Geometry check sheet. Reference: the model listing, model coordinates, mm. Face numbers are marked on the shaded views. A direction names the side the tool comes from. Round coordinates to 2 decimals unless told otherwise and drop trailing zeros. Order: outer loops, then holes, each group sorted by start corner. A loop starts at its lowest first (then second) coordinate and runs counter-clockwise, first axis right, second up. Notation, with made-up numbers: (70, 21) - (122, 21) arc R21 ccw to (122, 44) - close; hole circle Ø3 at (80, 40). An arc over 180 degrees is marked (long way). One line per question, with ' | ' between items. Start each with the question number.
Q1. Material ranges on line 1 along X through (y, z) = (-1.3, 1.25); line 2 along Z through (x, y) = (2.75, -1.25); line 3 along Z through (x, y) = (4.5, -0.45), recorded low to high.
Q2. Sectioned sample at C-C, the plane x = -0.5. Enter the section's corners in (y, z), then the cut area to 3 significant figures.
Q3. Sectioned sample at A-A, the plane y = -2. Enter the section's corners in (x, z), then the cut area to 3 significant figures.
Q4. Sectioned sample at B-B, the plane z = 2.25. Enter the section's corners in (x, y), then the cut area to 3 significant figures.
Q5. Tool access check on the marked faces 1 and 2. Record the directions out of +Z, -Z, +X, -X, +Y, -Y that give a thin tool (end or side, any length) a straight path to the whole face; none if there is none.
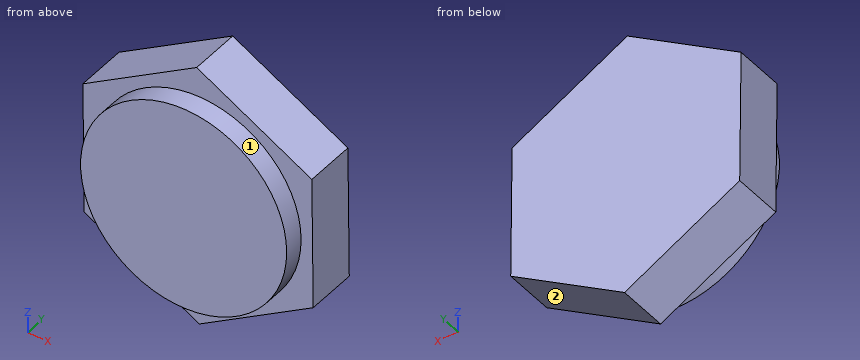
```python
from build123d import *

# Parameters (mm, degrees)
F1_DEPTH = 2.5
F2_R     = 5
F3_DEPTH = 3.5


with BuildPart() as f1:
    # F0 (on Front) → F1 (new body)
    with BuildSketch(Plane.XZ):
        Polygon((-0.067167, 6.41401), (-5.588279, 3.148836), (-5.521112, -3.265174), (0.067167, -6.41401), (5.588279, -3.148836), (5.521112, 3.265174), align=None)
    extrude(amount=F1_DEPTH)

    # F2 (on Front) → F3 (join)
    with BuildSketch(Plane.XZ):
        Circle(F2_R)
    extrude(amount=F3_DEPTH)


solid = f1.part
```
Determined:
1) line 1: x = -5.57 to 5.54 | line 2: z = -4.83 to 4.83 | line 3: z = -3.79 to 3.84
2) outline: (-3.5, -4.97) - (-2.5, -4.97) - (-2.5, -6.09) - (0, -6.09) - (0, 6.16) - (-2.5, 6.16) - (-2.5, 4.97) - (-3.5, 4.97) - close | area: 40.6 mm2
3) outline: (-5.59, 3.15) - (-5.52, -3.27) - (0.07, -6.41) - (5.59, -3.15) - (5.52, 3.27) - (-0.07, 6.41) - close | area: 107 mm2
4) outline: (-5.58, -2.5) - (-4.47, -2.5) - (-4.47, -3.5) - (4.47, -3.5) - (4.47, -2.5) - (5.53, -2.5) - (5.53, 0) - (-5.58, 0) - close | area: 36.7 mm2
5) face 1: -Y | face 2: -Z, +X, +Y, -Y
